```python
from build123d import *

# Parameters (mm, degrees)
SKETCH1_R               = 4.7625
BASIC_ROD_DEPTH         = 4.7625
BASIC_ROD_DEPTH_BACK    = 4.7625
THEX_DEPTH              = 4.7625
SKETCH2_R               = 1.89865
INTERNAL_CUT_DEPTH      = 5.7625
INTERNAL_CUT_DEPTH_BACK = 5.7625


with BuildPart() as part:
    # Sketch1 → Basic Rod (new body, two sides)
    with BuildSketch(Plane.XY) as basic_rod_sk:
        Circle(SKETCH1_R)
    extrude(amount=BASIC_ROD_DEPTH)
    extrude(basic_rod_sk.sketch, amount=-BASIC_ROD_DEPTH_BACK)

    # Sketch8 → THex (add, symmetric)
    with BuildSketch(Plane.XY):
        with BuildLine():
            Line((-0.742977689, 5.070302945), (-4.019522311, 3.178589026))
            ThreePointArc((-4.019522311, 3.178589026), (-4.43790388, 2.562225), (-4.7625, 1.891713919))
            Line((-4.7625, 1.891713919), (-4.7625, -1.891713919))
            ThreePointArc((-4.7625, -1.891713919), (-4.43790388, -2.562225), (-4.019522311, -3.178589026))
            Line((-4.019522311, -3.178589026), (-0.742977689, -5.070302945))
            ThreePointArc((-0.742977689, -5.070302945), (0, -5.12445), (0.742977689, -5.070302945))
            Line((0.742977689, -5.070302945), (4.019522311, -3.178589026))
            ThreePointArc((4.019522311, -3.178589026), (4.43790388, -2.562225), (4.7625, -1.891713919))
            Line((4.7625, -1.891713919), (4.7625, 1.891713919))
            ThreePointArc((4.7625, 1.891713919), (4.43790388, 2.562225), (4.019522311, 3.178589026))
            Line((4.019522311, 3.178589026), (0.742977689, 5.070302945))
            ThreePointArc((0.742977689, 5.070302945), (0, 5.12445), (-0.742977689, 5.070302945))
        make_face()
    extrude(amount=THEX_DEPTH, both=True)

    # Sketch2 → Internal Cut (cut, two sides)
    with BuildSketch(Plane.XY) as internal_cut_sk:
        Circle(SKETCH2_R)
    extrude(amount=INTERNAL_CUT_DEPTH, mode=Mode.SUBTRACT)
    extrude(internal_cut_sk.sketch, amount=-INTERNAL_CUT_DEPTH_BACK, mode=Mode.SUBTRACT)


solid = part.part
```
Build history of the part. All positions in model axes, mm. Coordinates: 2 decimals unless noted, no trailing zeros. Order: outer loops, then holes, each group sorted by start corner. A loop starts at its lowest first (then second) coordinate and runs counter-clockwise, first axis right, second up.
Item 1: Saw through at B-B on y = 0. List the corners of the cut face in (x, z), then the cut area to 3 significant figures.
Filled in:
outline: (-4.76, -4.76) - (-1.9, -4.76) - (-1.9, 4.76) - (-4.76, 4.76) - close; (1.9, -4.76) - (4.76, -4.76) - (4.76, 4.76) - (1.9, 4.76) - close
area: 54.6 mm2
Item 2: Drop a flat-ended pin along its axis: pin 1 Ø3 at (x, z) = (3, 3) entering from -Y. Give the stop position or say it passes through.
Filled in:
pin 1: stops at y = -4.63
Item 3: Saw through at A-A on z = -2.25. List the corners of the cut face in (x, y).
Filled in:
outline: (-4.76, -1.89) arc R5.12 ccw to (-4.02, -3.18) - (-0.74, -5.07) arc R5.12 ccw to (0.74, -5.07) - (4.02, -3.18) arc R5.12 ccw to (4.76, -1.89) - (4.76, 1.89) arc R5.12 ccw to (4.02, 3.18) - (0.74, 5.07) arc R5.12 ccw to (-0.74, 5.07) - (-4.02, 3.18) arc R5.12 ccw to (-4.76, 1.89) - close; hole circle Ø3.8 at (0, 0)
Item 4: Mould opens along X. For faces 1 (the flat face through (2.404, 4.111, 0.067)), 2 (the cylindrical face through (1.8, 0.6, 0.1)), 3 (the cylindrical face through (-0.01, -5.124, 0.067)), 4 (the flat face through (-2.404, -4.111, 0.067)) say: released by +X, released by -X, zero draft, split by the parting line, or undercut.
Filled in:
face 1: released by +X
face 2: undercut
face 3: split by the parting line
face 4: released by -X
Item 5: Saw through at C-C on x = 0. List the corners of the cut face in (y, z).
Filled in:
outline: (-5.12, -4.76) - (-1.9, -4.76) - (-1.9, 4.76) - (-5.12, 4.76) - close; (1.9, -4.76) - (5.12, -4.76) - (5.12, 4.76) - (1.9, 4.76) - close
Item 6: Saw through at D-D on x = 2.5. List the corners of the cut face in (y, z), then the cut area to 3 significant figures.
Filled in:
outline: (-4.06, -4.76) - (4.06, -4.76) - (4.06, 4.76) - (-4.06, 4.76) - close
area: 77.3 mm2
Item 7: Drill centre lines: L1, parallel to X at y = 0, z = -2.25; L2, parallel to X at y = 1.5, z = 3.5; L3, parallel to Y at x = 1, z = 3.5. Where is each one in solid material? Low to high.
Filled in:
L1: x = -4.76 to -1.9, 1.9 to 4.76
L2: x = -4.76 to -1.16, 1.16 to 4.76
L3: y = -4.92 to -1.61, 1.61 to 4.92
